from build123d import *

# Parameters (mm, degrees)
BASE_FLANGE1_DEPTH           = 3.175
EDGE_FLANGE1_DEPTH           = 16.378
EDGE_FLANGE2_STRIP_W         = 14.1732
EDGE_FLANGE2_STRIP_H         = 3.175
EDGE_FLANGE2_STRIP_CUT_DEPTH = 16.378
EDGE_FLANGE2_DEPTH           = 16.378
M5_CLEARANCE_HOLE1_D         = 5.5
M6_CLEARANCE_HOLE1_D         = 6.6
FILLET1_R                    = 2.54


# Sheet-metal steps are written as plain solids
with BuildPart() as part:
    # Sketch1 → Base-Flange1 (new body)
    with BuildSketch(Plane.XY):
        Polygon((40.772, -29.184600001), (40.772, -45.562600001), (40.772, -62.123600001), (-25.39999999, -62.123600001), (-25.39999999, -78.501600001), (57.15000001, -78.501600001), (57.15000001, -45.562600001), (61.9125, -45.562600001), (61.9125, -29.184600001), align=None)
    extrude(amount=-BASE_FLANGE1_DEPTH)

    # Edge-Flange1 section (across the edge) → Edge-Flange1 (add)
    with BuildSketch(Plane(origin=(62.6491, -45.562600001, 0), x_dir=(-1, 0, 0), z_dir=(0, 1, 0))):
        with BuildLine():
            Line((-3.175, 0.7366), (-3.175, 23.9268))
            Line((-3.175, 23.9268), (0, 23.9268))
            Line((0, 23.9268), (0, 0.7366))
            ThreePointArc((0, 0.7366), (0.215745145, 0.215745145), (0.7366, 0))
            Line((0.7366, 0), (0.7366, -3.175))
            ThreePointArc((0.7366, -3.175), (-2.029318885, -2.029318885), (-3.175, 0.7366))
        make_face()
    extrude(amount=EDGE_FLANGE1_DEPTH)

    # Edge-Flange2 strip (across the edge) → Edge-Flange2 strip cut (cut)
    with BuildSketch(Plane(origin=(65.8241, -29.184600001, 23.9268), x_dir=(0, 0, -1), z_dir=(0, -1, 0))):
        with Locations((-6.35, -1.5875)):
            Rectangle(EDGE_FLANGE2_STRIP_W, EDGE_FLANGE2_STRIP_H)
    extrude(amount=EDGE_FLANGE2_STRIP_CUT_DEPTH, mode=Mode.SUBTRACT)

    # Edge-Flange2 section (across the edge) → Edge-Flange2 (add)
    with BuildSketch(Plane(origin=(65.8241, -29.184600001, 23.9268), x_dir=(0, 0, -1), z_dir=(0, -1, 0))):
        with BuildLine():
            Line((-3.175, 0.7366), (-3.175, 60.325))
            Line((-3.175, 60.325), (0, 60.325))
            Line((0, 60.325), (0, 0.7366))
            ThreePointArc((0, 0.7366), (0.215745145, 0.215745145), (0.7366, 0))
            Line((0.7366, 0), (0.7366, -3.175))
            ThreePointArc((0.7366, -3.175), (-2.029318885, -2.029318885), (-3.175, 0.7366))
        make_face()
    extrude(amount=EDGE_FLANGE2_DEPTH)

    # M5 Clearance Hole1 (through all)
    with Locations(Plane.XY.offset(27.1018)):
        with Locations((119.7991, -37.373600001)):
            Hole(M5_CLEARANCE_HOLE1_D / 2)

    # M6 Clearance Hole1 (through all)
    with Locations(Plane.XY):
        with Locations((-17.0119, -70.312600001)):
            Hole(M6_CLEARANCE_HOLE1_D / 2)

    # Fillet1
    fillet1_edges = [part.edges().sort_by_distance(p)[0] for p in [
        (-25.39999999, -62.123600001, -1.5875),
        (40.772, -62.123600001, -1.5875),
        (40.772, -29.184600001, -1.5875),
        (57.15000001, -45.562600001, -1.5875),
        (57.15000001, -78.501600001, -1.5875),
        (-25.39999999, -78.501600001, -1.5875),
        (126.1491, -29.184600001, 25.5143),
        (126.1491, -45.562600001, 25.5143),
    ]]
    fillet(fillet1_edges, radius=FILLET1_R)


solid = part.part
Work out the finished part from the listing and answer in its coordinate system (mm). A direction names the side the tool comes from. Round coordinates to 2 decimals unless told otherwise and drop trailing zeros. Write each loop counter-clockwise with the first axis right and the second up, starting at its lowest first coordinate (ties: lowest second). Pieces come first, ordered by that corner, then holes.
1) Straight lines are drawn through the part: line 1 (Z direction, x = 111, y = -42); line 2 (X direction, y = -38.5, z = 24.5); line 3 (Z direction, x = 40, y = -67) (3 decimals). For each, find the intervals that lie inside material, in ascending order.
2) The mould has two halves that part along Y. Classify faces 1 (the flat face through (8, -62.124, -2)), 2 (the cylindrical face through (56.426, -77.738, -1.61)), 3 (the cylindrical face through (122.546, -37.253, 25.492)): pulls with the +Y half, pulls with the -Y half, needs draft (parallel to the pull), parting line crosses it, or undercut.
3) A cutting plane is placed at B-B (x = 101.5). Give the vertices of the cut face in (y, z), plus the area to 3 significant figures.
4) A tool of negligible diameter and unlimited length cuts with its end or side. For faces 4 (the flat face through (65.824, -37, 12)), 5 (the flat face through (62.649, -37, 12)), 6 (the flat face through (57.15, -62, -2)), 7 (the flat face through (74.7, -29.185, 24.2)), from which of +Z, -Z, +X, -X, +Y, -Y can it reach the whole face along a straight path? Write none if from no direction.
5) Given pin 1 Ø6 at (y, z) = (-39, 19.5) entering from +X; pin 2 Ø5 at (x, y) = (96, -33.5) entering from -Z; pin 3 Ø13 at (y, z) = (-40.5, 9.5) entering from -X, each flat-ended and moving along its own axis, determine where each tip first touches the part or whether it passes through.
6) A cutting plane is placed at A-A (z = 11.5). Give the vertices of the cut face in (x, y).
Completed:
1. line 1: z = 23.93 to 27.1
1. line 2: x = 62.87 to 117.29, 122.31 to 126.15
1. line 3: z = -3.175 to 0
2. face 1: pulls with the +Y half
2. face 2: pulls with the -Y half
2. face 3: undercut
3. outline: (-45.56, 23.93) - (-29.18, 23.93) - (-29.18, 27.1) - (-45.56, 27.1) - close
3. area: 52.0 mm2
4. face 4: -Z, +X, +Y, -Y
4. face 5: +Z, -X, +Y, -Y
4. face 6: +Z, -Z, +X, -Y
4. face 7: +Z, -Z, +X, -X, +Y
5. pin 1: stops at x = 65.82
5. pin 2: stops at z = 23.93
5. pin 3: stops at x = 62.65
6. outline: (62.65, -45.56) - (65.82, -45.56) - (65.82, -29.18) - (62.65, -29.18) - close
